from build123d import *

# Parameters (mm, degrees)
F2_R = 1


# Not quite as in the source:
# - a feature names something its author has since deleted; it is built from what else it names


with BuildPart() as f3:
    # F3: sweep along a path in F0
    with BuildLine(Plane.XY) as f3_path:
        Line((-73.4692310878, 100), (-73.4692310878, 92))
        ThreePointArc((-73.4692310878, 92), (-72.8834446502, 90.5857864376), (-71.4692310878, 90))
        Line((-71.4692310878, 90), (-70.4692310878, 90))
        ThreePointArc((-70.4692310878, 90), (-69.0550175254, 90.5857864376), (-68.4692310878, 92))
        Line((-68.4692310878, 92), (-68.4692310878, 98))
        ThreePointArc((-68.4692310878, 98), (-67.8834446502, 99.4142135624), (-66.4692310878, 100))
        Line((-66.4692310878, 100), (-65.4692310878, 100))
        ThreePointArc((-65.4692310878, 100), (-64.0550175254, 99.4142135624), (-63.4692310878, 98))
        Line((-63.4692310878, 98), (-63.4692310878, 5))
        ThreePointArc((-63.4692310878, 5), (-64.9336971819, 1.4644660941), (-68.4692310878, 0))
        Line((-68.4692310878, 0), (-73.4692310878, 0))
    # F2 (on plane+point) → F3 (sweep)
    with BuildSketch(Plane.XZ.offset(-100)):
        with Locations((-73.4692310878, 0)):
            Circle(F2_R)
    sweep(path=f3_path.line)


solid = f3.part
Can you work these out from the model? Positions are in its coordinate system, mm. A direction names the side the tool comes from. Coordinates: 2 decimals unless noted, no trailing zeros. Loops run counter-clockwise (first coordinate to the right, second up) from the corner with the lowest first, then second, coordinate; pieces in that order, holes last. Notation, with made-up numbers: (89, 57.25) - (146, 57.25) arc R31 ccw to (146, 81.25) - close; hole circle Ø10 at (4.5, 44.5). An arc over 180 degrees is marked (long way). Answer as a JSON object with one key per item and string values. Group by question number.
Item 1: If we section it at A-A (z = 0): List the corners of the cut face in (x, y) for me, plus the area to 3 significant figures.
Item 2: On a 3-axis mill with a long thin cutter (end or side, diameter ignored), from which of +Z, -Z, +X, -X, +Y, -Y can I reach the whole of each face in a straight line? I mean faces 1 (the face through (-64.47, 50.85, 0.04)), 2 (the face through (-73.469, 0, 0)), 3 (the face through (-71, 0, -1)). Say none if no direction works.
Item 3: If I drill on L1, parallel to X at y = 91.5, z = 0.4; L2, parallel to X at y = 52, z = -0.1; L3, parallel to Y at x = -69.75, z = -0.6, over which ranges is the centre line in solid material (lowest first)? Write a range as from..to.
Item 4: If we mould it in two halves opening along Y, with no side actions, what happens to faces 4 (the face through (-71, 89, 0)), 5 (the face through (-73, 100, 0)), 6 (the face through (-74.47, 95.94, 0.04))? For each: released by +Y, released by -Y, zero draft, split by the parting line, or undercut.
Item 5: For pin 1 (0.6 mm diameter, centred on x = -73.5, z = 0, fed in from +Y); pin 2 (1.5 mm diameter, centred on x = -64, y = 90.5, fed in from -Z), each with a flat end and sliding along its axis, tell me the tip position at first contact or that it passes through.
Item 6: If we section it at B-B (y = 45.5): List the corners of the cut face in (x, z) for me.
Returned:
{
 "1": {"outline": "(-74.47, 92) arc R3 ccw to (-71.47, 89) - (-70.47, 89) arc R3 ccw to (-67.47, 92) - (-67.47, 98) arc R1 cw to (-66.47, 99) - (-65.47, 99) arc R1 cw to (-64.47, 98) - (-64.47, 5) arc R4 cw to (-68.47, 1) - (-73.47, 1) - (-73.47, -1) - (-68.47, -1) arc R6 ccw to (-62.47, 5) - (-62.47, 98) arc R3 ccw to (-65.47, 101) - (-66.47, 101) arc R3 ccw to (-69.47, 98) - (-69.47, 92) arc R1 cw to (-70.47, 91) - (-71.47, 91) arc R1 cw to (-72.47, 92) - (-72.47, 100) - (-74.47, 100) - close", "area": "269 mm²"},
 "2": {"face 1": "none", "face 2": "+Z, -Z, -X, -Y", "face 3": "-X"},
 "3": {"L1": "x = -74.34..-72.43, -69.51..-67.6, -64.39..-62.55", "L2": "x = -64.46..-62.47", "L3": "y = -0.8..0.8, 89.29..91.04"},
 "4": {"face 4": "undercut", "face 5": "released by +Y", "face 6": "zero draft"},
 "5": {"pin 1": "stops at y = 100", "pin 2": "stops at z = -1"},
 "6": {"outline": "circle Ø2 at (-63.47, 0)"}
}
